Could you check a few things on this model? Use its own coordinates, in mm. A direction names the side the tool comes from. Coordinates: 2 decimals unless noted, no trailing zeros. Order: outer loops, then holes, each group sorted by start corner. A loop starts at its lowest first (then second) coordinate and runs counter-clockwise, first axis right, second up. Notation, with made-up numbers: (-16.5, 76.5) -> (37.5, 76.5) arc R3 ccw to (37.5, 80.5) -> close; hole circle Ø8 at (11, 66.25). An arc over 180 degrees is marked (long way). Put each result on its own line as item: value. Start each with the question number.
Q1. Will these pins go through, and if not, where does the flat tip stop? pin 1 (3 mm diameter, centred on x = -25.5, z = 197.5, fed in from -Y); pin 2 (2 mm diameter, centred on x = 19.5, z = 405, fed in from -Y); pin 3 (3 mm diameter, centred on y = 99.5, z = 636.5, fed in from +X).
Q2. For faces 1 (the face through (-39, 120, 0)), 2 (the face through (42, 105.702, 493)), which set-ups out of +Z, -Z, +X, -X, +Y, -Y let a thin tool reach every point of the face, with its end or its side?
Q3. Please list where these lines run through material, in increasing order: line 1 along Y through (x, z) = (6, 931); line 2 along X through (y, z) = (105, 298); line 3 along Y through (x, z) = (22, 321).
Q4. If we section it at A-A (z = 224.5): Please give me the cut outline in (x, y).
Q5. If we section it at B-B (x = -5.5): Please give me the cut outline in (y, z), and give its area (3 significant figures).
from build123d import *

# Parameters (mm, degrees)
F1_DEPTH = 1000


with BuildPart() as f1:
    # F0 (on Top) → F1 (new body)
    with BuildSketch(Plane.XY):
        with BuildLine():
            Line((51.771715, 105.701796), (51.771715, 165.701796))
            Line((51.771715, 165.701796), (-95.728285, 165.701796))
            Line((-95.728285, 165.701796), (-95.728285, 45.701796))
            Line((-95.728285, 45.701796), (-45.728285, 45.701796))
            Line((-45.728285, 45.701796), (-45.728285, 60.701796))
            Line((-45.728285, 60.701796), (-30.728285, 60.701796))
            ThreePointArc((-30.728285, 60.701796), (-20.477022, 85.450533), (4.271715, 95.701796))
            Line((4.271715, 95.701796), (4.271715, 105.701796))
            Line((4.271715, 105.701796), (14.271715, 105.701796))
            Line((14.271715, 105.701796), (14.271715, 115.701796))
            Line((14.271715, 115.701796), (21.771715, 115.701796))
            ThreePointArc((21.771715, 115.701796), (28.842783, 112.772864), (31.771715, 105.701796))
            Line((31.771715, 105.701796), (51.771715, 105.701796))
        make_face()
    extrude(amount=F1_DEPTH)


solid = f1.part
The answers:
1. pin 1: y = 76.42
1. pin 2: y = 115.7
1. pin 3: x = 4.27
2. face 1: -Z, +X, -X, +Y, -Y
2. face 2: +Z, -Z, +X, -Y
3. line 1: 105.7 to 165.7
3. line 2: -95.73 to 4.27
3. line 3: 115.7 to 165.7
4. outline: (-95.73, 45.7) -> (-45.73, 45.7) -> (-45.73, 60.7) -> (-30.73, 60.7) arc R35 cw to (4.27, 95.7) -> (4.27, 105.7) -> (14.27, 105.7) -> (14.27, 115.7) -> (21.77, 115.7) arc R10 cw to (31.77, 105.7) -> (51.77, 105.7) -> (51.77, 165.7) -> (-95.73, 165.7) -> close
5. outline: (94.31, 0) -> (165.7, 0) -> (165.7, 1000) -> (94.31, 1000) -> close
5. area: 71,400 mm^2
